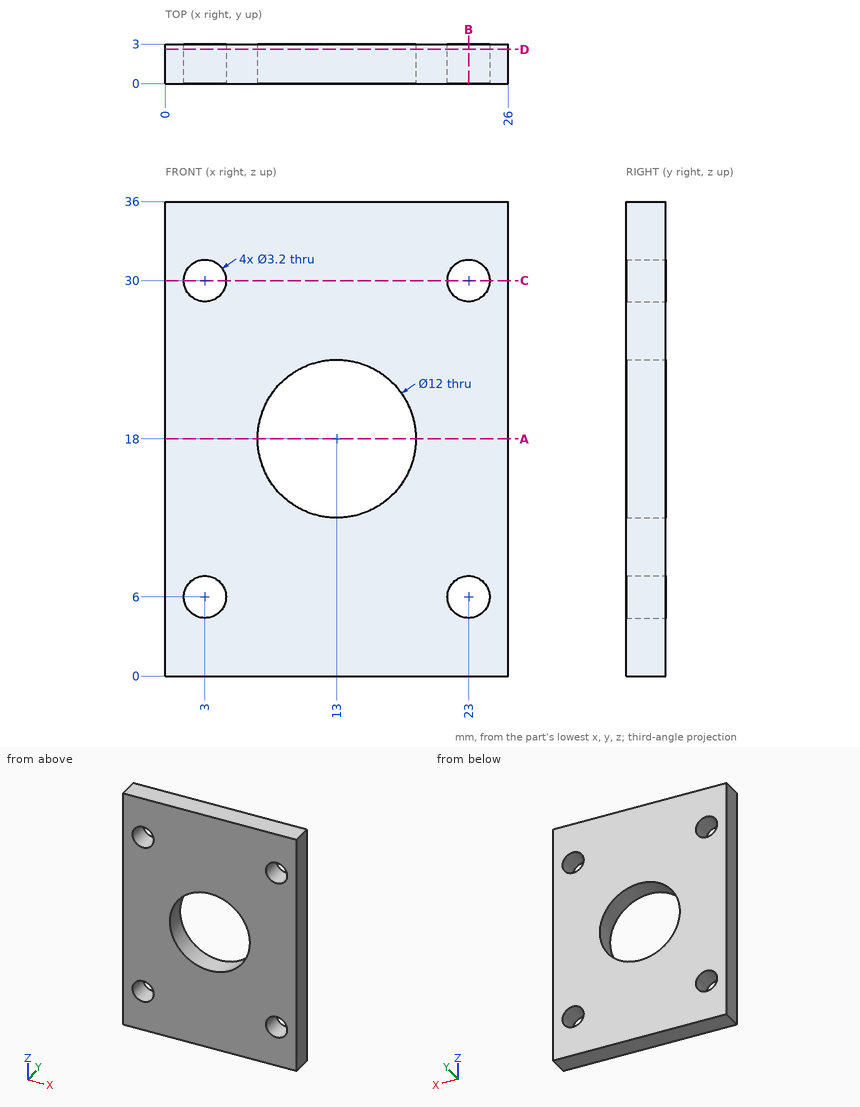
Answer from the drawing. Dimensions are ordinates in mm from the lowest x, y and z of the part. Give positions to 0.01 mm unless a question says otherwise; leave off trailing zeros. Order: outer loops, then holes, each group sorted by start corner. A loop starts at its lowest first (then second) coordinate and runs counter-clockwise, first axis right, second up. Notation, with made-up numbers: (67.5, -3) - (97.5, -3) arc R29 ccw to (97.5, 21) - close; hole circle Ø4 at (-37, 78.5). An arc over 180 degrees is marked (long way). One line per item, written item: value. Start each with the question number.
1. Consider line 1 (Z direction, x = 3, y = 2.1); line 2 (X direction, y = 2.15, z = 30); line 3 (X direction, y = 2, z = 18). Determine where each line is inside the solid, lowest interval first.
2. Section B-B, the plane x = 23 is taken. Write down the section's boundary in (y, z).
3. Section A-A, the plane z = 18 is taken. Write down the section's boundary in (x, y).
4. Section D-D, the plane y = 2.6 is taken. Write down the section's boundary in (x, z), then the cut area to 3 significant figures.
5. Section C-C, the plane z = 30 is taken. Write down the section's boundary in (x, y).
Filled sheet:
1. line 1: 0 to 4.4, 7.6 to 28.4, 31.6 to 36
1. line 2: 0 to 1.4, 4.6 to 21.4, 24.6 to 26
1. line 3: 0 to 7, 19 to 26
2. outline: (0, 0) - (3, 0) - (3, 4.4) - (0, 4.4) - close; (0, 7.6) - (3, 7.6) - (3, 28.4) - (0, 28.4) - close; (0, 31.6) - (3, 31.6) - (3, 36) - (0, 36) - close
3. outline: (0, 0) - (7, 0) - (7, 3) - (0, 3) - close; (19, 0) - (26, 0) - (26, 3) - (19, 3) - close
4. outline: (0, 0) - (26, 0) - (26, 36) - (0, 36) - close; hole circle Ø3.2 at (3, 6); hole circle Ø3.2 at (3, 30); hole circle Ø12 at (13, 18); hole circle Ø3.2 at (23, 6); hole circle Ø3.2 at (23, 30)
4. area: 791 mm²
5. outline: (0, 0) - (1.4, 0) - (1.4, 3) - (0, 3) - close; (4.6, 0) - (21.4, 0) - (21.4, 3) - (4.6, 3) - close; (24.6, 0) - (26, 0) - (26, 3) - (24.6, 3) - close
